from build123d import *

# Parameters (mm, degrees)
BOSS_EXTRUDE1_DEPTH = 8
BOSS_EXTRUDE2_DEPTH = 8
BOSS_EXTRUDE3_DEPTH = 16
SKETCH4_R           = 2.165
CUT_EXTRUDE1_DEPTH  = 48.748826419
CUT_EXTRUDE2_DEPTH  = 8


with BuildPart() as part:
    # Sketch1 → Boss-Extrude1 (new body)
    with BuildSketch(Plane.XY):
        with BuildLine():
            Line((-19.5, 13.830605225), (-19.5, 0))
            Line((-19.5, 0), (-28.9068116, 0))
            ThreePointArc((-28.9068116, 0), (0, 28.9068116), (28.9068116, 0))
            Line((28.9068116, 0), (23.9068116, 0))
            ThreePointArc((23.9068116, 0), (7.257851427, 22.778481809), (-19.5, 13.830605225))
        make_face()
    extrude(amount=BOSS_EXTRUDE1_DEPTH)

    # Sketch2 → Boss-Extrude2 (add)
    with BuildSketch(Plane.XY.offset(8)):
        with BuildLine():
            Line((-28.9068116, 0), (-18.11056, 0))
            ThreePointArc((-18.11056, 0), (0, 18.11056), (18.11056, 0))
            Line((18.11056, 0), (28.9068116, 0))
            ThreePointArc((28.9068116, 0), (0, 28.9068116), (-28.9068116, 0))
        make_face()
    extrude(amount=BOSS_EXTRUDE2_DEPTH)

    # Sketch3 → Boss-Extrude3 (add, through all)
    with BuildSketch(Plane.XY.offset(16)):
        with BuildLine():
            Line((-28.9068116, 0), (-38.11056, 0))
            Line((-38.11056, 0), (-38.11056, 5))
            Line((-38.11056, 5), (-28.471103893, 5))
            ThreePointArc((-28.471103893, 5), (-28.797678666, 2.509474109), (-28.9068116, 0))
        make_face()
    extrude(amount=-BOSS_EXTRUDE3_DEPTH)

    # Sketch4 → Cut-Extrude1 (cut, through all)
    with BuildSketch(Plane(origin=(0, 5, 0), x_dir=(1, 0, 0), z_dir=(0, 1, 0))):
        with Locations(Location((-33.290831946, -8, 0), (0, 0, 180))):
            Circle(SKETCH4_R)
    extrude(amount=-CUT_EXTRUDE1_DEPTH, mode=Mode.SUBTRACT)

    # Sketch5 → Cut-Extrude2 (cut)
    with BuildSketch(Plane(origin=(0, 0, 0), x_dir=(-1, 0, 0), z_dir=(0, 0, -1))):
        Polygon((0, 0), (-17.347099568, 16.450342776), (-43.024104882, 25.187540913), (-58.13318285, -8.31229871), align=None)
    extrude(amount=-CUT_EXTRUDE2_DEPTH, mode=Mode.SUBTRACT)


solid = part.part
Model file for the job. Use its own axes, mm. A direction names the side the tool comes from. Round coordinates to 2 decimals unless told otherwise and drop trailing zeros. Order: outer loops, then holes, each group sorted by start corner. A loop starts at its lowest first (then second) coordinate and runs counter-clockwise, first axis right, second up.
(1) Band-saw the part on D-D (x = 11). List the corners of the cut face in (y, z).
(2) Band-saw the part on B-B (x = 0). List the corners of the cut face in (y, z).
(3) Band-saw the part on C-C (x = -29.5). List the corners of the cut face in (y, z).
(4) Drill centre lines: line 1 (X direction, y = 19.75, z = 0.5); line 2 (Y direction, x = -32, z = 11); line 3 (Z direction, x = 20.5, y = 14). Where is each one in solid material? Low to high.
(5) Band-saw the part on A-A (z = 2.75). List the corners of the cut face in (x, y), then the cut area to 3 significant figures.
(6) Pin check, flat tips, straight feed: pin 1 (4 mm diameter, centred on x = -2.5, z = 9, fed in from +Y); pin 2 (12 mm diameter, centred on x = -3.5, y = 13, fed in from -Z); pin 3 (2 mm diameter, centred on x = -7, z = 8, fed in from -Y). Stop position of each tip, or through.
(7) 3-axis set-ups, long thin cutter, end or side, ignore diameter. For faces 1 (the face through (19.87, 17.31, 3.94)), 2 (the face through (-1.401, 23.866, 3.944)), 3 (the face through (-6.366, 28.197, 7.888)), 4 (the face through (-36, 5, 8)): which of +Z, -Z, +X, -X, +Y, -Y reach the whole face in a straight line?
(8) Pull direction Z, two halves, no side cores. Call faces 5 (the face through (-12, 21, 0)), 6 (the face through (-35.356, 2.535, 8.65)), 7 (the face through (-0.398, 18.106, 11.944)): released by +Z, released by -Z, zero draft, split by the parting line, or undercut.
Verdict:
1. outline: (14.39, 8) - (21.23, 8) - (21.23, 0) - (26.73, 0) - (26.73, 16) - (14.39, 16) - close
2. outline: (18.11, 8) - (23.91, 8) - (23.91, 0) - (28.91, 0) - (28.91, 16) - (18.11, 16) - close
3. outline: (0, 0) - (5, 0) - (5, 16) - (0, 16) - close
4. line 1: x = -21.11 to -13.47, 13.47 to 21.11
4. line 2: y = 0 to 5
4. line 3: z = 8 to 16
5. outline: (-38.11, 0) - (-19.5, 0) - (-19.5, 13.83) arc R23.91 cw to (17.35, 16.45) - (22.46, 18.19) arc R28.91 ccw to (-28.47, 5) - (-38.11, 5) - close
5. area: 408 mm2
6. pin 1: stops at y = 28.9
6. pin 2: stops at z = 8
6. pin 3: stops at y = 16.25
7. face 1: -Z, +X, -Y
7. face 2: -Z, -Y
7. face 3: +Z, -Z, +Y
7. face 4: +Z, -Z, -X, +Y
8. face 5: released by -Z
8. face 6: undercut
8. face 7: zero draft
